Here's how the part is built. I have some questions about the finished solid (model axes, mm). A direction names the side the tool comes from. Coordinates: 2 decimals unless noted, no trailing zeros. Write each loop counter-clockwise with the first axis right and the second up, starting at its lowest first coordinate (ties: lowest second). Pieces come first, ordered by that corner, then holes.
Item 1: If we mould it in two halves opening along X, with no side actions, what happens to faces 5 (the face through (134, -10, -1)), 6 (the face through (143.231, 0, -14.6)), 7 (the face through (0, 0, 0)), 8 (the face through (133.938, 0.126, 7.885))? For each: pulls with the +X half, pulls with the -X half, needs draft (parallel to the pull), parting line crosses it, or undercut.
Item 2: I want a section at A-A (z = 0). Please give me the cut outline in (x, y).
Item 3: I'm going to push flat-ended pins straight in: P1, Ø5.5, axis at x = 132.5, z = 10.5, coming from the +Y side; P2, Ø2, axis at x = 91.5, z = -4, coming from the -Y side; P3, Ø3.5, axis at x = 136, z = 10.5, coming from the -Y side; P4, Ø3, axis at x = 134.81, z = -4.91, coming from the -Y side. Where does each tip first touch, or does it pass through?
Item 4: For faces 1 (the face through (134, 0, -15)), 2 (the face through (133, 10, -1)), 3 (the face through (64, 0, 6)), 4 (the face through (135, 0, -14)), which set-ups out of +Z, -Z, +X, -X, +Y, -Y let a thin tool reach every point of the face, with its end or its side?
Item 5: I want a section at B-B (y = 0). Please give me the cut outline in (x, z), and give its area (3 significant figures).
Item 6: I want a section at D-D (z = 11). Count the separate pieces of the cut face and the enclosed holes in it, and give its area (3 significant figures).
Item 7: Please list where these lines run through material, in increasing order: line 1 (X direction, y = 5, z = -11); line 2 (X direction, y = -1, z = 8); line 3 (X direction, y = 7, z = 9).
Item 8: I want a section at C-C (x = 30). Please give me the cut outline in (y, z), and give its area (3 significant figures).
Autodesk Inventor part; units mm, degrees
ref_plane "YZ Plane" through (0, 0, 0) normal (1, 0, 0) x (0, 1, 0)
ref_plane "XZ Plane" through (0, 0, 0) normal (0, 1, 0) x (-1, 0, 0)
ref_plane "XY Plane" through (0, 0, 0) normal (0, 0, 1) x (1, 0, 0)
sketch "Sketch1" plane through (0, 0, 0) normal (1, 0, 0) x (0, 1, 0)
  circle A0 centre (0, 0) radius 25
  dimension "d0" = 50
extrude "Extrusion1" add sketch "Sketch1" along normal blind 5
fillet "Fillet1" radius 2 1 edges at (5, -25, 0)
sketch "Sketch2" plane through (5, 0, 0) normal (1, 0, 0) x (0, 0, -1)
  circle A0 centre (0, 0) radius 6
  dimension "d4" = 12
extrude "Extrusion2" add sketch "Sketch2" along normal blind 120
sketch "Sketch3" plane through (125, 0, 0) normal (1, 0, 0) x (0, 0, -1)
  line L0 (15, 10) -> (-15, 10)
  line L1 (-15, 10) -> (-15, -10)
  line L2 (-15, -10) -> (15, -10)
  line L3 (15, -10) -> (15, 10)
  point P0 (0, 0)
  dimension "d7" = 20
  dimension "d8" = 30
  dimension "d9" = 15
  dimension "d10" = 10
extrude "Extrusion3" add sketch "Sketch3" along normal blind 20
sketch "Sketch4" plane through (145, 0, 0) normal (1, 0, 0) x (0, 0, -1)
  line L0 (-14, -9) -> (14, -9)
  line L1 (14, -9) -> (14, 9)
  line L2 (14, 9) -> (-14, 9)
  line L3 (-14, 9) -> (-14, -9)
  line L4 (-15, -10) -> (15, -10)
  line L5 (15, -10) -> (15, 10)
  point P0 (0, 0)
  dimension "d13" = 28
  dimension "d14" = 18
  dimension "d15" = 1
  dimension "d16" = 1
extrude "Extrusion4" cut sketch "Sketch4" against normal blind 19
sketch "Sketch5" plane through (125, 10, 15) normal (0, 1, 0) x (1, 0, 0)
  line L0 (0, 0) -> (20, 0)
  line L1 (2.7176, 0) -> (1.4771, 2.1348)
  line L2 (1.4771, 2.1348) -> (16.6105, 12.2356)
  line L3 (16.6105, 12.2356) -> (18.2313, 9.8073)
  line L4 (18.2313, 9.8073) -> (18.2313, 30)
  line L5 (0, 30) -> (20, 30)
  line L6 (20, 30) -> (20, 0)
  line L7 (20, 30) -> (20, 0)
  line L8 (20, 0) -> (2.7176, 0)
  point P0 (-125, 15)
extrude "Extrusion5" cut sketch "Sketch5" against normal blind 30
sketch "Sketch6" plane through (141.6105, 9, 2.7644) normal (0.5551496, 0, 0.8317505) x (0.8317505, 0, -0.5551496)
  line L0 (-18.1947, 1) -> (0, 1)
  line L1 (0, -19) -> (-18.1947, -19)
  line L2 (0, 1) -> (-18.1947, 1)
  line L3 (-18.1947, 1) -> (-18.1947, -19)
  line L4 (-18.1947, -19) -> (0, -19)
  line L5 (0, -19) -> (0, 1)
  point P0 (-116.25, -9)
extrude "Extrusion6" add sketch "Sketch6" along normal blind 0.5
sketch "Sketch7" plane through (125, -10, -15) normal (0, -1, 0) x (1, 0, 0)
  circle A0 centre (9.8115, 10.087) radius 2.5
  point P0 (-125, 15)
  dimension "d23" = 5
extrude "Extrusion7" cut sketch "Sketch7" against normal blind 25
sketch "Sketch8" plane through (143.2313, -10, 5.1927) normal (-0.8317505, 0, 0.5551496) x (0.5551496, 0, 0.8317505)
  line L0 (-16.7953, 0) -> (0, 0)
  line L1 (0, 20) -> (-16.7953, 20)
  line L2 (0, 0) -> (-2.3419, 0)
  line L3 (-2.3419, 0) -> (-2.3419, 20)
  line L4 (-2.3419, 20) -> (0, 20)
  line L5 (0, 20) -> (0, 0)
  point P0 (-83.8338, 10)
  point P1 (-2.3419, 0)
extrude "Extrusion8" add sketch "Sketch8" along normal blind 1
sketch "Sketch9" plane through (141.8881, 9, 3.1803) normal (0.5551496, 0, 0.8317505) x (0.8317505, 0, -0.5551496)
  line L0 (-18.1947, -19) -> (-18.3481, -19)
  line L1 (-18.1947, -18) -> (0, -18)
  line L2 (-18.1947, -19) -> (-0.9871, -19)
  line L3 (-0.9871, -19) -> (-0.9871, -18)
  line L4 (-0.9871, -18) -> (-18.1947, -18)
  line L5 (-18.1947, -18) -> (-18.1947, -19)
  point P0 (-116.25, -9)
  point P1 (-18.1947, -18)
extrude "Extrusion9" add sketch "Sketch9" along normal blind 2
sketch "Sketch10" plane through (141.8881, 9, 3.1803) normal (0.5551496, 0, 0.8317505) x (0.8317505, 0, -0.5551496)
  line L0 (-18.1947, 1) -> (-18.1947, -18)
  line L1 (1.107, 0) -> (-3.893, 0)
  line L2 (-18.1947, 1) -> (-0.936, 1)
  line L3 (-0.936, 1) -> (-0.936, 0)
  line L4 (-0.936, 0) -> (-18.1947, 0)
  line L5 (-18.1947, 0) -> (-18.1947, 1)
  point P0 (-116.25, -9)
  point P1 (-3.893, 0)
extrude "Extrusion10" add sketch "Sketch10" along normal blind 2
properties part number "reception robot design"
Answer:
1. face 5: needs draft
1. face 6: pulls with the +X half
1. face 7: pulls with the -X half
1. face 8: undercut
2. outline: (0, -25) - (3, -25) arc R2 ccw to (5, -23) - (5, -6) - (125, -6) - (125, -10) - (143.23, -10) - (143.23, -9) - (126, -9) - (126, 9) - (143.23, 9) - (143.23, 10) - (125, 10) - (125, 6) - (5, 6) - (5, 23) arc R2 ccw to (3, 25) - (0, 25) - close
3. P1: stops at y = 10
3. P2: stops at y = -5.2
3. P3: stops at y = -10
3. P4: passes through
4. face 1: -Z, +X, +Y, -Y
4. face 2: +Z, -Z, +X, +Y
4. face 3: none
4. face 4: +X
5. outline: (0, -25) - (3, -25) arc R2 ccw to (5, -23) - (5, -6) - (125, -6) - (125, -15) - (143.23, -15) - (143.23, -14) - (126, -14) - (126, 14) - (127.14, 14) - (127.72, 15) - (125, 15) - (125, 6) - (5, 6) - (5, 23) arc R2 ccw to (3, 25) - (0, 25) - close; (126.48, 12.87) - (141.61, 2.76) - (141.89, 3.18) - (126.75, 13.28) - close; (141.1, 3.8) - (141.93, 3.24) - (143.23, 5.19) - (142.4, 5.75) - close
5. area: 1,750 mm2
6. separate pieces: 2
6. enclosed holes: 1
6. area: 274 mm2
7. line 1: x = 0 to 5, 125 to 126
7. line 2: x = 0 to 5, 125 to 126, 133.77 to 134.67
7. line 3: x = 0 to 5, 125 to 126, 132.27 to 133.17
8. outline: circle Ø12 at (0, 0)
8. area: 113 mm2
